Autodesk Inventor part; units mm, degrees
ref_plane "YZ Plane" through (0, 0, 0) normal (1, 0, 0) x (0, 1, 0)
ref_plane "XZ Plane" through (0, 0, 0) normal (0, 1, 0) x (-1, 0, 0)
ref_plane "XY Plane" through (0, 0, 0) normal (0, 0, 1) x (1, 0, 0)
ref_plane "Work Plane13" through (0, 3, 0) normal (0, 1, 0) x (1, 0, 0)
sketch "Sketch45" plane through (0, 3, 0) normal (0, 1, 0) x (1, 0, 0)
  line L0 (35, -20) -> (-3, -20)
  line L1 (-3, -20) -> (-3, 20)
  line L2 (-3, 20) -> (35, 20)
  line L3 (35, 20) -> (35, -20)
  point P0 (0, 0)
  dimension "d142" = 38
  dimension "d143" = 40
extrude "Extrusion34" add sketch "Sketch45" along normal blind 30
sketch "Sketch46" plane through (0, 33, 0) normal (0, 1, 0) x (1, 0, 0)
  point P0 (0, 0)
ref_plane "Work Plane11" through (0, 0, 0) normal (0, -1, 0) x (1, 0, 0)
sketch "Sketch47" plane through (0, 0, 0) normal (0, -1, 0) x (1, 0, 0)
  circle A0 centre (16, 0) radius 18
  point P0 (0, 0)
  dimension "d146" = 36
extrude "Extrusion35" cut sketch "Sketch47" against normal blind 30 draft -15
sketch "Sketch48" plane through (0, 33, 0) normal (0, 1, 0) x (1, 0, 0)
  point P0 (0, 0)
sketch "Sketch49" plane through (0, 33, 0) normal (0, 1, 0) x (1, 0, 0)
  circle A0 centre (20, 0) radius 1
  point P0 (0, 0)
  dimension "d149" = 2
extrude "Extrusion36" cut sketch "Sketch49" against normal through all
ref_plane "Work Plane7" through (35, 3, -20) normal (0, 0, -1) x (-1, 0, 0)
sketch "Sketch58" plane through (35, 3, -20) normal (0, 0, -1) x (-1, 0, 0)
  line L0 (7, 20) -> (27, 20)
  line L1 (27, 20) -> (27, 5)
  line L2 (27, 5) -> (7, 5)
  line L3 (7, 5) -> (7, 20)
  point P0 (35, -3)
  dimension "d156" = 20
  dimension "d157" = 15
extrude "Extrusion38" cut sketch "Sketch58" against normal blind 15
ref_plane "Work Plane4" through (-3, 3, -20) normal (-1, 0, 0) x (0, 0, 1)
sketch "Sketch59" plane through (-3, 3, -20) normal (-1, 0, 0) x (0, 0, 1)
  line L0 (4, 25) -> (8, 25)
  line L1 (8, 25) -> (8, 5)
  line L2 (8, 5) -> (4, 5)
  line L3 (4, 5) -> (4, 25)
  point P0 (20, -3)
  dimension "d160" = 4
  dimension "d161" = 20
extrude "Extrusion39" cut sketch "Sketch59" against normal blind 35
ref_plane "Work Plane1" through (0, 3, 0) normal (0, 1, 0) x (1, 0, 0)
ref_plane "Work Plane6" through (0, 23, 0) normal (0, 1, 0) x (1, 0, 0)
sketch "Sketch62" plane through (-3, 3, -20) normal (-1, 0, 0) x (0, 0, 1)
  circle A0 centre (20, 15) radius 3.5
  point P0 (20, -3)
  dimension "d172" = 7
extrude "Extrusion42" cut sketch "Sketch62" against normal through all
sketch "Sketch65" plane through (0, 3, 0) normal (0, -1, 0) x (1, 0, 0)
  line L0 (-3, -12) -> (32, -12)
  line L1 (28, -20) -> (28, -16)
  line L2 (3.5815, -12) -> (28, -12)
  line L3 (28, -12) -> (28, -17.2375)
  line L4 (28, -17.2375) -> (3.5815, -17.2375)
  line L5 (3.5815, -17.2375) -> (3.5815, -12)
  point P0 (0, 0)
extrude "Extrusion44" add sketch "Sketch65" against normal blind 5
properties part number "liquid port_only_v04"
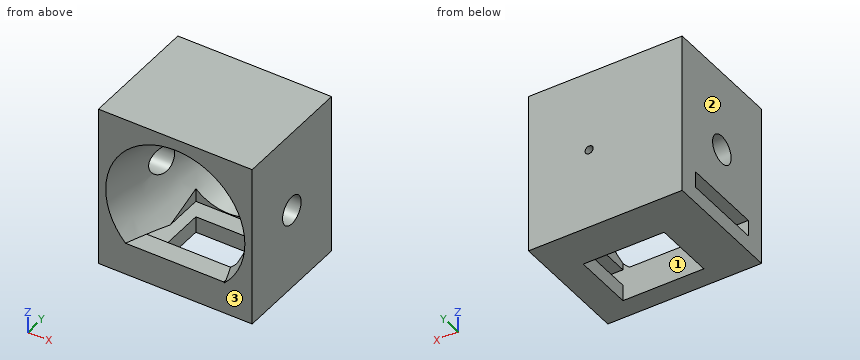
Design review of the part built by this model. Coordinates are the model's own, in mm. Face numbers are marked on the shaded views. Round coordinates to 2 decimals unless told otherwise and drop trailing zeros. Write each loop counter-clockwise with the first axis right and the second up, starting at its lowest first coordinate (ties: lowest second). Pieces come first, ordered by that corner, then holes.
Item 1: We need section A-A on z = 0. Write out the cut boundary in (x, y).
Item 2: We need section D-D on y = 18. Write out the cut boundary in (x, z).
Item 3: Clearance check with flat-ended pins moving along their axes: pin 1 Ø10 at (x, z) = (11.5, -1) entering from -Y; pin 2 Ø1.2 at (y, z) = (20, -14) entering from -X. State where each tip first meets the part, or that it passes through.
Item 4: For probe 1 along Z at (x, y) = (1, 18); probe 2 along X at (y, z) = (31, 0); probe 3 along Z at (x, y) = (20, 31.7), list the stretches that pass through material, from the lowest coordinate up.
Item 5: The part is to be moulded in two halves that separate along X. For the marked faces 1, 2 and 3, say which applies: +X half, -X half, draft (parallel to the pull), parting line (faces both ways), or undercut.
Item 6: We need section C-C on y = 25. Write out the cut boundary in (x, z), and give its area (3 significant figures).
Item 7: We need section B-B on x = 16. Write out the cut boundary in (y, z).
Returned:
1. outline: (-3, 3) - (-1.2, 3) - (1.89, 14.5) - (-3, 14.5) - close; (-3, 21.5) - (3.76, 21.5) - (6.04, 30) - (19, 30) - (19, 33) - (-3, 33) - close; (21, 30) - (25.96, 30) - (28.24, 21.5) - (35, 21.5) - (35, 33) - (21, 33) - close; (30.11, 14.5) - (33.2, 3) - (35, 3) - (35, 14.5) - close
2. outline: (-3, -20) - (8, -20) - (8, -16) - (-3, -16) - close; (-3, -12) - (8, -12) - (8, -10.47) arc R13.18 cw to (3.3, -3.5) - (-3, -3.5) - close; (-3, 3.5) - (3.3, 3.5) arc R13.18 cw to (28.7, 3.5) - (35, 3.5) - (35, 20) - (-3, 20) - close; (28, -20) - (35, -20) - (35, -3.5) - (28.7, -3.5) arc R13.18 cw to (28, -5.44) - (28, -12) - (32, -12) - (32, -16) - (28, -16) - close
3. pin 1: stops at y = 30
3. pin 2: stops at x = 32
4. probe 1: z = -20 to -16, -12 to -3.5, 3.5 to 20
4. probe 2: x = -3 to 19, 21 to 35
4. probe 3: z = -20 to -1, 1 to 20
5. face 1: undercut
5. face 2: -X half
5. face 3: draft
6. outline: (-3, -20) - (35, -20) - (35, 20) - (-3, 20) - (-3, -12) - (32, -12) - (32, -16) - (-3, -16) - close; hole circle Ø22.6 at (16, 0)
6. area: 979 mm2
7. outline: (3, -20) - (8, -20) - (8, -12) - (3, -12) - close; (3, 17.2) - (30, 9.96) - (30, -9.96) - (23, -11.84) - (23, -12) - (28, -12) - (28, -16) - (23, -16) - (23, -20) - (33, -20) - (33, 20) - (3, 20) - close
